from build123d import *

# Parameters (mm, degrees)
SKETCH1_W           = 38.1
SKETCH1_H           = 2
BOSS_EXTRUDE1_DEPTH = 3
CHAMFER1_SIZE       = 0.1
CHAMFER2_SIZE       = 0.1


with BuildPart() as part:
    # Sketch1 → Revolve1 (revolve)
    with BuildSketch(Plane.XY, mode=Mode.PRIVATE) as revolve1_sk:
        with Locations((19.05, 1)):
            Rectangle(SKETCH1_W, SKETCH1_H)
    revolve(revolve1_sk.sketch.rotate(Axis((-15.554693394, 0, 0), (1, 0, 0)), 90), axis=Axis((-15.554693394, 0, 0), (1, 0, 0)))

    # Sketch2 → Boss-Extrude1 (add)
    with BuildSketch(Plane.ZY):
        Polygon((0, 4.041451884), (-3.5, 2.020725942), (-3.5, -2.020725942), (0, -4.041451884), (3.5, -2.020725942), (3.5, 2.020725942), align=None)
    extrude(amount=BOSS_EXTRUDE1_DEPTH)

    # Chamfer1
    chamfer1_edges = [part.edges().sort_by_distance(p)[0] for p in [
        (0, 3.031088913, -1.75),
        (0, 0, -3.5),
        (0, -3.031088913, -1.75),
        (0, -3.031088913, 1.75),
        (0, 0, 3.5),
        (-3, 3.031088913, 1.75),
        (-3, 3.031088913, -1.75),
        (-3, 0, -3.5),
        (-3, -3.031088913, -1.75),
        (-3, -3.031088913, 1.75),
        (-3, 0, 3.5),
        (0, 3.031088913, 1.75),
    ]]
    chamfer(chamfer1_edges, length=CHAMFER1_SIZE)

    # Chamfer2
    chamfer2_edges = [part.edges().sort_by_distance(p)[0] for p in [
        (38.1, 0, -2),
    ]]
    chamfer(chamfer2_edges, length=CHAMFER2_SIZE)


solid = part.part
Read the model definition and answer for the solid it produces. Units are mm, in the model's axes. A direction names the side the tool comes from. Give positions to 0.01 mm unless a question says otherwise; leave off trailing zeros. Write each loop counter-clockwise with the first axis right and the second up, starting at its lowest first coordinate (ties: lowest second). Pieces come first, ordered by that corner, then holes. Notation, with made-up numbers: (4, 35.25) -> (46, 35.25) arc R20 cw to (46, 67.25) -> close; hole circle Ø7 at (-38.5, 35.25). An arc over 180 degrees is marked (long way). Answer as a JSON object with one key per item and string values. Group by question number.
1) Each of these flat-tipped pins is pushed along its axis until it touches: P1, Ø4, axis at x = 21.5, z = 0.5, coming from the +Y side; P2, Ø1.5, axis at x = 15, y = 0, coming from the -Z side; P3, Ø1, axis at x = 15, y = -1.5, coming from the -Z side. Where does it stop, or does it pass through?
2) Find section C-C (x = 15). Write down the section's boundary in (y, z), and give its area (3 significant figures).
3) Consider L1, parallel to X at y = -3.5, z = 0.5; L2, parallel to Z at x = 28.5, y = -1; L3, parallel to Z at x = 35, y = 0.75. Determine where each line is inside the solid, lowest interval first. Write a range as from..to.
4) A tool of negligible diameter and unlimited length cuts with its end or side. For faces 1 (the cylindrical face through (19, 2, 0)), 2 (the flat face through (-1.5, -3, -1.8)), from which of +Z, -Z, +X, -X, +Y, -Y can it reach the whole face along a straight path? Write none if from no direction.
5) Find section B-B (z = 2.75). Write down the section's boundary in (x, y).
6) Find section D-D (y = -3.5). Write down the section's boundary in (x, z), and give its area (3 significant figures).
7) Find section A-A (y = 0). Write down the section's boundary in (x, z).
Values follow:
{
 "1": {"P1": "stops at y = 2", "P2": "stops at z = -2", "P3": "stops at z = -1.73"},
 "2": {"outline": "circle Ø4 at (0, 0)", "area": "12.6 mm2"},
 "3": {"L1": "x = -3..0", "L2": "z = -1.73..1.73", "L3": "z = -1.85..1.85"},
 "4": {"face 1": "+X", "face 2": "-Z, +X, -X, -Y"},
 "5": {"outline": "(-3, -2.34) -> (-2.9, -2.45) -> (-0.1, -2.45) -> (0, -2.34) -> (0, 2.34) -> (-0.1, 2.45) -> (-2.9, 2.45) -> (-3, 2.34) -> close"},
 "6": {"outline": "(-3, -0.74) -> (-2.9, -0.94) -> (-0.1, -0.94) -> (0, -0.74) -> (0, 0.74) -> (-0.1, 0.94) -> (-2.9, 0.94) -> (-3, 0.74) -> close", "area": "5.59 mm2"},
 "7": {"outline": "(-3, -3.4) -> (-2.9, -3.5) -> (-0.1, -3.5) -> (0, -3.4) -> (0, -2) -> (38, -2) -> (38.1, -1.9) -> (38.1, 1.9) -> (38, 2) -> (0, 2) -> (0, 3.4) -> (-0.1, 3.5) -> (-2.9, 3.5) -> (-3, 3.4) -> close"}
}
